```python
from build123d import *

# Parameters (mm, degrees)
SKETCH1_W           = 42
SKETCH1_H           = 42
BOSS_EXTRUDE3_DEPTH = 2
SKETCH1_26_W        = 46
SKETCH1_26_H        = 2
SKETCH1_26_W_2      = 2
SKETCH1_26_H_2      = 46
BOSS_EXTRUDE6_DEPTH = 13


with BuildPart() as part:
    # Sketch1 → Boss-Extrude3 (new body)
    with BuildSketch(Plane(origin=(0, 0, 0), x_dir=(1, 0, 0), z_dir=(0, 1, 0))):
        Polygon((-42, 31), (-44, 29), (-44, -17), (-42, -19), (4, -19), (6, -17), (6, 29), (4, 31), align=None)
        with Locations((-19, 6)):
            Rectangle(SKETCH1_W, SKETCH1_H, mode=Mode.SUBTRACT)
    extrude(amount=BOSS_EXTRUDE3_DEPTH)

    # Sketch1_26 → Boss-Extrude6 (add)
    with BuildSketch(Plane(origin=(0, 0, 0), x_dir=(1, 0, 0), z_dir=(0, 1, 0))):
        with Locations((-19, -20)):
            Rectangle(SKETCH1_26_W, SKETCH1_26_H)
        with Locations((-19, 32)):
            Rectangle(SKETCH1_26_W, SKETCH1_26_H)
        with Locations((7, 6)):
            Rectangle(SKETCH1_26_W_2, SKETCH1_26_H_2)
        with Locations((-45, 6)):
            Rectangle(SKETCH1_26_W_2, SKETCH1_26_H_2)
    extrude(amount=BOSS_EXTRUDE6_DEPTH)


solid = part.part
```
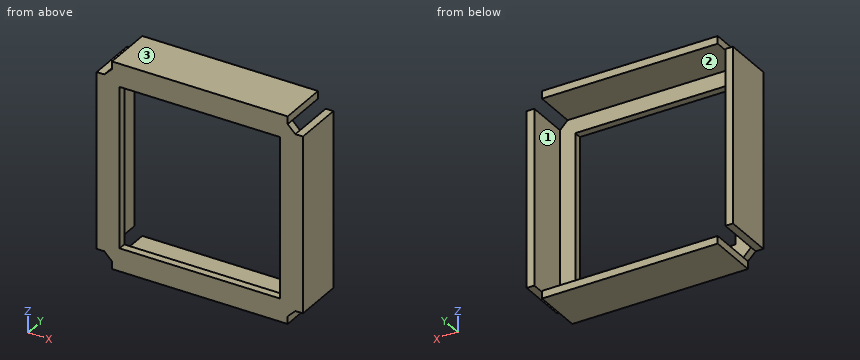
Read the model definition and answer for the solid it produces. Units are mm, in the model's axes. Face numbers are marked on the shaded views. Coordinates: 2 decimals unless noted, no trailing zeros. Loops run counter-clockwise (first coordinate to the right, second up) from the corner with the lowest first, then second, coordinate; pieces in that order, holes last. Notation, with made-up numbers: (-26.5, 85) -> (8.5, 85) arc R30 ccw to (8.5, 111) -> close; hole circle Ø5 at (68.5, 4.5). An arc over 180 degrees is marked (long way). Return JSON: item names as keys, results as strings.
Item 1: Find section B-B (y = 1). Determine the outline of the cut face in (x, z).
Answers:
{"outline": "(-46, -29) -> (-44, -29) -> (-42, -31) -> (-42, -33) -> (4, -33) -> (4, -31) -> (6, -29) -> (8, -29) -> (8, 17) -> (6, 17) -> (4, 19) -> (4, 21) -> (-42, 21) -> (-42, 19) -> (-44, 17) -> (-46, 17) -> close; hole (-40, -27) -> (2, -27) -> (2, 15) -> (-40, 15) -> close"}
Item 2: Find the intervals of material crossed by probe 1 along Z at (x, y) = (-11, 10.75); probe 2 along X at (y, z) = (10.75, -0.5); probe 3 along Z at (x, y) = (-30, 0.75), in increasing order.
Answers:
{"probe 1": "z = -33 to -31, 19 to 21", "probe 2": "x = -46 to -44, 6 to 8", "probe 3": "z = -33 to -27, 15 to 21"}
Item 3: Flat-ended cylindrical pins translate along their axes: P1, Ø2, axis at x = 7, y = 7, coming from the +Z side; P2, Ø1, axis at x = 7, y = 5, coming from the -Z side; P3, Ø1, axis at y = 6, z = -32, coming from the -X side; P4, Ø2, axis at x = -0.5, z = 8.5, coming from the -Y side (3 decimals). Find the tip coordinate at first contact, or state that the pin passes through.
Answers:
{"P1": "stops at z = 17", "P2": "stops at z = -29", "P3": "stops at x = -42", "P4": "passes through"}
Item 4: For a pull along Z with two mould halves and no side action, classify the marked faces 1, 2 and 3 as +Z half, -Z half, draft (parallel to the pull), parting line (faces both ways), or undercut.
Answers:
{"face 1": "draft", "face 2": "undercut", "face 3": "+Z half"}
Item 5: Find section D-D (y = 11). Determine the outline of the cut face in (x, z).
Answers:
{"outline": "(-46, -29) -> (-44, -29) -> (-44, 17) -> (-46, 17) -> close; (-42, -33) -> (4, -33) -> (4, -31) -> (-42, -31) -> close; (-42, 19) -> (4, 19) -> (4, 21) -> (-42, 21) -> close; (6, -29) -> (8, -29) -> (8, 17) -> (6, 17) -> close"}
Item 6: Find section A-A (x = -7). Determine the outline of the cut face in (y, z), plus the area to 3 significant figures.
Answers:
{"outline": "(0, -33) -> (13, -33) -> (13, -31) -> (2, -31) -> (2, -27) -> (0, -27) -> close; (0, 15) -> (2, 15) -> (2, 19) -> (13, 19) -> (13, 21) -> (0, 21) -> close", "area": "68.0 mm2"}
Item 7: Find section C-C (z = 11). Determine the outline of the cut face in (x, y), plus the area to 3 significant figures.
Answers:
{"outline": "(-46, 0) -> (-40, 0) -> (-40, 2) -> (-44, 2) -> (-44, 13) -> (-46, 13) -> close; (2, 0) -> (8, 0) -> (8, 13) -> (6, 13) -> (6, 2) -> (2, 2) -> close", "area": "68.0 mm2"}
